from build123d import *

# Parameters (mm, degrees)
BASE_SKETCH_W                   = 90
BASE_SKETCH_H                   = 60
BASE_EXTRUDE_DEPTH              = 5
CRADLE_SKETCH_W                 = 20
CRADLE_SKETCH_H                 = 60
CRADLE_EXTRUDE_DEPTH            = 25
NO_6_MOUNTING_HOLES_D           = 3.7973
NO_6_MOUNTING_HOLES_CSINK_D     = 7.0866
NO_6_MOUNTING_HOLES_CSINK_ANGLE = 82
MOVE_START                      = 15
MOVE_FACE_OUTLINE_W             = 20
MOVE_FACE_OUTLINE_H             = 60
MOVE_FACE_DEPTH                 = 10
CLAMP_THREADED_HOLE_D           = 2.5
CRADLE_FILLETS_R                = 6
BASE_FILLETS_R                  = 6


# Read off the part's stored shape, not the designer's step: Move Face
with BuildPart() as part:
    # Base Sketch → Base Extrude (new body)
    with BuildSketch(Plane.XY):
        with Locations((-2.5, 0)):
            Rectangle(BASE_SKETCH_W, BASE_SKETCH_H)
    extrude(amount=BASE_EXTRUDE_DEPTH)

    # Cradle Sketch → Cradle Extrude (add)
    with BuildSketch(Plane.XY):
        with Locations((-32.6, 0)):
            Rectangle(CRADLE_SKETCH_W, CRADLE_SKETCH_H)
        with Locations((32.6, 0)):
            Rectangle(CRADLE_SKETCH_W, CRADLE_SKETCH_H)
    extrude(amount=CRADLE_EXTRUDE_DEPTH)

    # No. 6 Mounting Holes (through all)
    with Locations(Plane.XY.offset(5)):
        with Locations((-15.1, 20), (15.1, 20), (-15.1, -20), (15.1, -20)):
            CounterSinkHole(NO_6_MOUNTING_HOLES_D / 2, NO_6_MOUNTING_HOLES_CSINK_D / 2, counter_sink_angle=NO_6_MOUNTING_HOLES_CSINK_ANGLE)

    # Pump and Motor Revolve Cut Sketch → Pump and Motor Revolve Cut (revolve, cut)
    with BuildSketch(Plane(origin=(0, 0, 0), x_dir=(1, 0, 0), z_dir=(0, 1, 0))):
        Polygon((-44, -33.5), (-44, -3), (2, -3), (2, -14.25), (66, -14.25), (66, -33.5), align=None)
    revolve(axis=Axis((66, 0, 33.5), (-1, 0, 0)), mode=Mode.SUBTRACT)

    # Move Face outline → Move Face (cut)
    with BuildSketch(Plane.XY.offset(MOVE_START)):
        with Locations((-32.6, 0)):
            Rectangle(MOVE_FACE_OUTLINE_W, MOVE_FACE_OUTLINE_H)
    extrude(amount=MOVE_FACE_DEPTH, mode=Mode.SUBTRACT)

    # Clamp Threaded Hole (through all)
    with Locations(Plane.XY.offset(25)):
        with Locations((32.6, -26.5)):
            clamp_threaded_hole = Hole(CLAMP_THREADED_HOLE_D / 2)

    # Threaded Hole Mirror: Clamp Threaded Hole across plane
    add(clamp_threaded_hole.mirror(Plane.ZX), mode=Mode.SUBTRACT)

    # Cradle Fillets
    cradle_fillets_edges = [part.edges().sort_by_distance(p)[0] for p in [
        (-42.6, 30, 10),
        (42.6, 30, 12.5),
        (42.6, -30, 12.5),
        (-42.6, -30, 10),
        (22.6, 30, 15),
        (22.6, -30, 15),
        (-22.6, 30, 10),
        (-22.6, -30, 10),
    ]]
    fillet(cradle_fillets_edges, radius=CRADLE_FILLETS_R)

    # Base Fillets
    base_fillets_edges = [part.edges().sort_by_distance(p)[0] for p in [
        (-47.5, -30, 2.5),
        (-47.5, 30, 2.5),
    ]]
    fillet(base_fillets_edges, radius=BASE_FILLETS_R)


solid = part.part
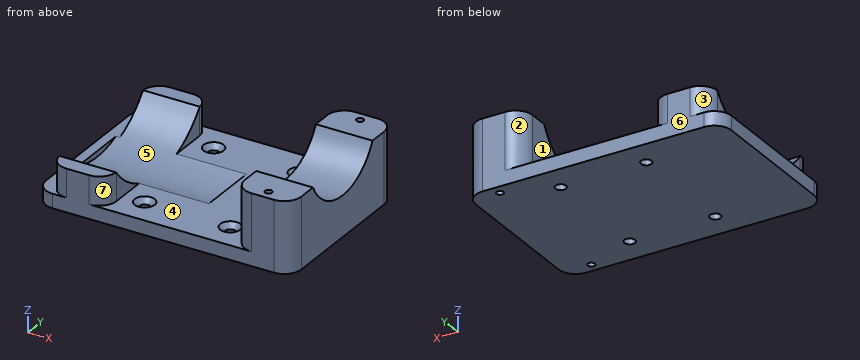
Read the model definition and answer for the solid it produces. Units are mm, in the model's axes. Face numbers are marked on the shaded views. A direction names the side the tool comes from. Give positions to 0.01 mm unless a question says otherwise; leave off trailing zeros. Loops run counter-clockwise (first coordinate to the right, second up) from the corner with the lowest first, then second, coordinate; pieces in that order, holes last. Notation, with made-up numbers: (-33, 84) - (-6, 84) arc R30 cw to (-6, 120) - close; hole circle Ø3 at (86.25, -0.5). An arc over 180 degrees is marked (long way). Answer as CSV lines item,"result". Start each with the question number.
1) Find section A-A (x = -15.1). Write down the section's boundary in (y, z), then the cut area to 3 significant figures.
2) Find section B-B (z = 17.75). Write down the section's boundary in (x, y), then the cut area to 3 significant figures.
3) Which of the six approach directions +Z, -Z, +X, -X, +Y, -Y give full straight-line access (tool end or side, diameter ignored) to the marked faces 1, 2 and 3?
4) Determine the mould class of the marked faces 4, 5, 6 and 7 for opening direction Y: released by +Y, released by -Y, zero draft, split by the parting line, or undercut.
5) Find section C-C (y = 20). Write down the section's boundary in (x, z).
6) Each of these flat-tipped pins is pushed along its axis until it touches: pin 1 Ø5 at (y, z) = (-17.5, 8.5) entering from -X; pin 2 Ø1.7 at (x, y) = (-29, 28) entering from +Z; pin 3 Ø4.5 at (x, y) = (-15.1, 20) entering from +Z. Where does it stop, or does it pass through?
7) Find section D-D (z = 7.25). Write down the section's boundary in (x, y), then the cut area to 3 significant figures.
8) Straight lines are drawn through the part: L1, parallel to Y at x = 15.1, z = 1.65; L2, parallel to X at y = -20, z = 2.45; L3, parallel to Y at x = 32.6, z = 7.25. For each, find the intervals that lie inside material, in ascending order. Write a range as from..to.
Findings below:
1,outline,"(-30, 0) - (-21.9, 0) - (-21.9, 3.11) - (-23.54, 5) - (-30, 5) - close; (-18.1, 0) - (18.1, 0) - (18.1, 3.11) - (16.46, 5) - (10.86, 5) arc R30.5 cw to (-10.86, 5) - (-16.46, 5) - (-18.1, 3.11) - close; (21.9, 0) - (30, 0) - (30, 5) - (23.54, 5) - (21.9, 3.11) - close"
1,area,"227 mm^2"
2,outline,"(22.6, -24) arc R6 ccw to (28.6, -30) - (36.6, -30) arc R6 ccw to (42.6, -24) - (42.6, -11.07) - (22.6, -11.07) - close; (22.6, 11.07) - (42.6, 11.07) - (42.6, 24) arc R6 ccw to (36.6, 30) - (28.6, 30) arc R6 ccw to (22.6, 24) - close; hole circle Ø2.5 at (32.6, -26.5); hole circle Ø2.5 at (32.6, 26.5)"
2,area,"717 mm^2"
3,face 1,"+Z, +Y, -Y"
3,face 2,"+Z, +Y"
3,face 3,"+Z, -X, +Y"
4,face 4,"zero draft"
4,face 5,"undercut"
4,face 6,"released by +Y"
4,face 7,"released by -Y"
5,outline,"(-47.5, 0) - (-17, 0) - (-17, 3.11) - (-18.64, 5) - (-22.6, 5) - (-22.6, 10.47) - (-42.6, 10.47) - (-42.6, 5) - (-47.5, 5) - close; (-13.2, 0) - (13.2, 0) - (13.2, 3.11) - (11.56, 5) - (-11.56, 5) - (-13.2, 3.11) - close; (17, 0) - (42.6, 0) - (42.6, 25) - (22.6, 25) - (22.6, 5) - (18.64, 5) - (17, 3.11) - close"
6,pin 1,"x = -42.6"
6,pin 2,"z = 15"
6,pin 3,"z = 3.51"
7,outline,"(-42.6, -24) arc R6 ccw to (-36.6, -30) - (-28.6, -30) arc R6 ccw to (-22.6, -24) - (-22.6, -15.53) - (-42.6, -15.53) - close; (-42.6, 15.53) - (-22.6, 15.53) - (-22.6, 24) arc R6 ccw to (-28.6, 30) - (-36.6, 30) arc R6 ccw to (-42.6, 24) - close; (22.6, -24) arc R6 ccw to (28.6, -30) - (36.6, -30) arc R6 ccw to (42.6, -24) - (42.6, 24) arc R6 ccw to (36.6, 30) - (28.6, 30) arc R6 ccw to (22.6, 24) - close; hole circle Ø2.5 at (32.6, -26.5); hole circle Ø2.5 at (32.6, 26.5)"
7,area,"1,710 mm^2"
8,L1,"-30..-21.9, -18.1..18.1, 21.9..30"
8,L2,"-47.5..-17, -13.2..13.2, 17..42.6"
8,L3,"-30..-27.75, -25.25..25.25, 27.75..30"
